Source: CAD feature listing. Evaluate the final solid. Frame: model axes, mm. Face numbers are marked on the shaded views. A direction names the side the tool comes from. Round coordinates to 2 decimals unless told otherwise and drop trailing zeros. Write each loop counter-clockwise with the first axis right and the second up, starting at its lowest first coordinate (ties: lowest second). Pieces come first, ordered by that corner, then holes. Notation, with made-up numbers: M 13,87 L 59,87 A20 ccw 59,108 Z; hole C -18,50.25 d4. An arc over 180 degrees is marked long. Answer in a Markdown table with one row per item.
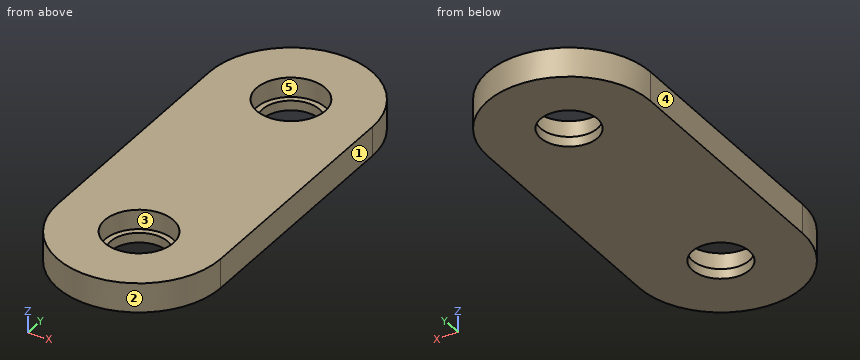
Autodesk Inventor part; units mm, degrees
ref_plane "YZ Plane" through (0, 0, 0) normal (1, 0, 0) x (0, 1, 0)
ref_plane "XZ Plane" through (0, 0, 0) normal (0, 1, 0) x (-1, 0, 0)
ref_plane "XY Plane" through (0, 0, 0) normal (0, 0, 1) x (1, 0, 0)
sketch "Szkic1" plane through (0, 0, 0) normal (0, 0, 1) x (1, 0, 0)
  line L0 (0, -75) -> (0, 75) construction
  line L1 (50, -75) -> (50, 75)
  line L2 (-50, 75) -> (-50, -75)
  arc A0 (-50, -75) -> (50, -75) centre (0, -75) ccw
  arc A1 (50, 75) -> (-50, 75) centre (0, 75) ccw
  point P0 (0, 0)
  dimension "d2" = 100
extrude "Wyciągnięcie proste2" add sketch "Szkic1" along normal blind 18
sketch "Szkic2" plane through (0, 0, 18) normal (0, 0, 1) x (1, 0, 0)
  circle A0 centre (0, 75) radius 21.05
  circle A1 centre (0, -75) radius 21.05
  point P0 (0, 0)
  dimension "d7" = 42.1
  dimension "d8" = 42.1
extrude "Wyciągnięcie proste3" cut sketch "Szkic2" against normal blind 12
sketch "Szkic3" plane through (0, -75, 6) normal (0, 0, 1) x (1, 0, 0)
  circle A0 centre (0, 0) radius 17.5
  point P0 (0, 75)
  dimension "d11" = 35
sketch "Szkic4" plane through (0, 75, 6) normal (0, 0, 1) x (1, 0, 0)
  circle A0 centre (0, 0) radius 17.5
  point P0 (0, -75)
  dimension "d12" = 35
extrude "Wyciągnięcie proste4" cut sketch "Szkic4" against normal blind 12
extrude "Wyciągnięcie proste5" cut sketch "Szkic3" against normal blind 12
equation "\"d12\" = d11"
properties part number "podstawa" material "MDF - płyta pilśniowa o średniej gęstości"
Q1. Section A-A (x = 0). Return loops of the section in (y, z), and give its area (3 significant figures).
Solutions:
| item | result |
|---|---|
| outline | M -125,0 L -92.5,0 L -92.5,6 L -96.05,6 L -96.05,18 L -125,18 Z; M -57.5,0 L 57.5,0 L 57.5,6 L 53.95,6 L 53.95,18 L -53.95,18 L -53.95,6 L -57.5,6 Z; M 92.5,0 L 125,0 L 125,18 L 96.05,18 L 96.05,6 L 92.5,6 Z |
| area | 3,070 mm2 |
Q2. Section C-C (y = 66). Return loops of the section in (x, z), and give its area (3 significant figures).
Solutions:
| item | result |
|---|---|
| outline | M -50,0 L -15.01,0 L -15.01,6 L -19.03,6 L -19.03,18 L -50,18 Z; M 15.01,0 L 50,0 L 50,18 L 19.03,18 L 19.03,6 L 15.01,6 Z |
| area | 1,160 mm2 |
Q3. Material intervals for probe 1 along Y at (x, z) = (0, 2.45); probe 2 along Y at (x, z) = (0, 11); probe 3 along Z at (x, y) = (15, 62), sorted ascending.
Solutions:
| item | result |
|---|---|
| probe 1 | y = -125 to -92.5, -57.5 to 57.5, 92.5 to 125 |
| probe 2 | y = -125 to -96.05, -53.95 to 53.95, 96.05 to 125 |
| probe 3 | z = 0 to 6 |
Q4. Pull-direction query (Y, two-part tool) for the marked faces 1, 2 and 3; classes: pulls with the +Y half, pulls with the -Y half, needs draft (parallel to the pull), parting line crosses it, or undercut.
Solutions:
| item | result |
|---|---|
| face 1 | needs draft |
| face 2 | pulls with the -Y half |
| face 3 | undercut |
Q5. Access query for the marked faces 4 and 5. Directions: +Z, -Z, +X, -X, +Y, -Y. A direction counts if a zero-diameter tool reaches every point of the face in a straight line with its end or side. Return the directions, or none.
Solutions:
| item | result |
|---|---|
| face 4 | +Z, -Z, -X, +Y, -Y |
| face 5 | +Z |
Q6. Section B-B (z = 8.75). Return loops of the section in (x, y).
Solutions:
| item | result |
|---|---|
| outline | M -50,-75 A50 ccw 50,-75 L 50,75 A50 ccw -50,75 Z; hole C 0,-75 d42.1; hole C 0,75 d42.1 |
Q7. Contact query for flat-ended pins moving along their axis: pin 1 Ø1.5 at (x, z) = (-12, 7.5) entering from +Y; pin 2 Ø3 at (x, z) = (-5, 4.5) entering from +Y; pin 3 Ø4 at (x, z) = (28, 6.5) entering from +Y. Output: stop coordinate, or through.
Solutions:
| item | result |
|---|---|
| pin 1 | stops at y = 123.72 |
| pin 2 | stops at y = 124.88 |
| pin 3 | stops at y = 117.71 |
Q8. Section D-D (x = 36). Return loops of the section in (y, z), and give its area (3 significant figures).
Solutions:
| item | result |
|---|---|
| outline | M -109.7,0 L 109.7,0 L 109.7,18 L -109.7,18 Z |
| area | 3,950 mm2 |
